The figure shows three views and two pictorial views of one solid part (mm, origin at its lowest corner). Answer the questions. Round coordinates to 2 decimals unless told otherwise and drop trailing zeros. Order: outer loops, then holes, each group sorted by start corner. A loop starts at its lowest first (then second) coordinate and runs counter-clockwise, first axis right, second up. Notation, with made-up numbers: M 48.5,-1.75 L 54.5,-1.75 A26 cw 54.5,30.25 Z; hole C -24.5,52 d3. An arc over 180 degrees is marked long. Return JSON: item names as keys, results as strings.
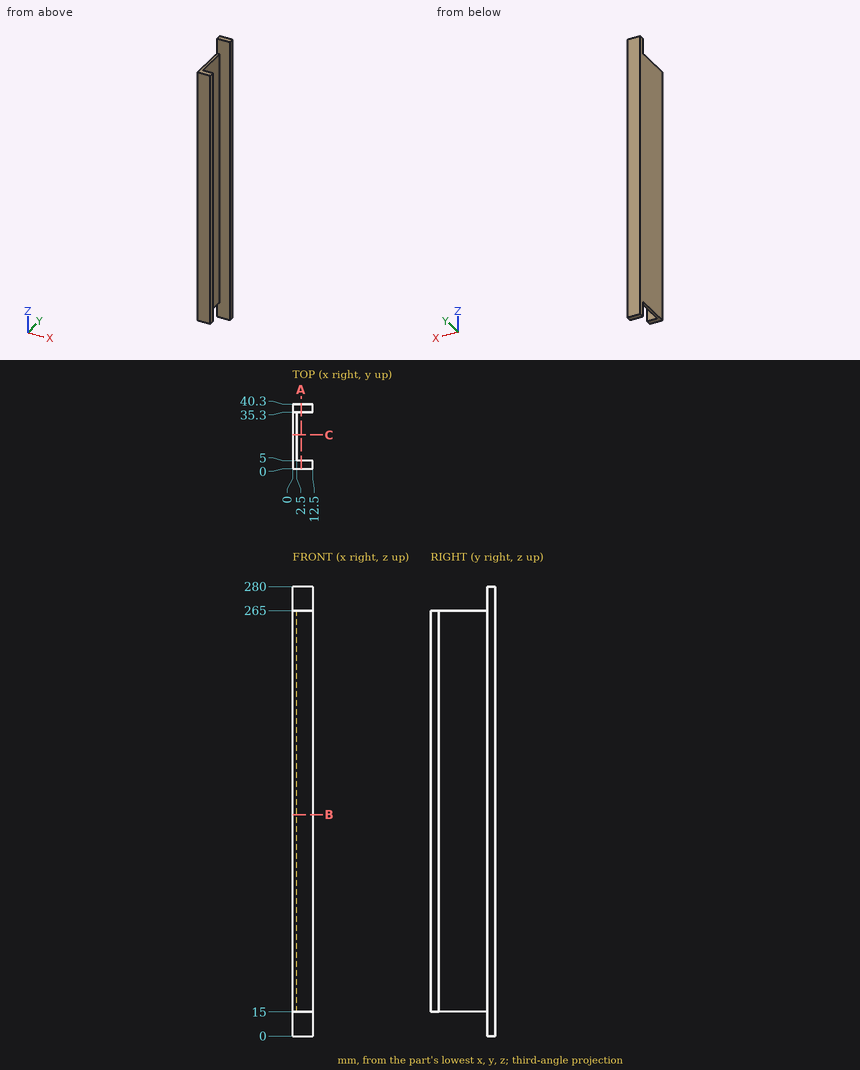
Item 1: Each of these flat-tipped pins is pushed along its axis until it touches: pin 1 (6 mm diameter, centred on y = 27.5, z = 212, fed in from -X); pin 2 (1.5 mm diameter, centred on x = 3.5, y = 28.5, fed in from +Z); pin 3 (10 mm diameter, centred on y = 29.5, z = 150.5, fed in from +X). Where does it stop, or does it pass through?
Output:
{"pin 1": "stops at x = 0", "pin 2": "passes through", "pin 3": "stops at x = 2.5"}
Item 2: Find section B-B (z = 138). Determine the outline of the cut face in (x, y), plus the area to 3 significant figures.
Output:
{"outline": "M 0,0 L 12.5,0 L 12.5,5 L 2.5,5 L 2.5,35.3 L 12.5,35.3 L 12.5,40.3 L 0,40.3 Z", "area": "201 mm^2"}
Item 3: Find section C-C (y = 21). Determine the outline of the cut face in (x, z), plus the area to 3 significant figures.
Output:
{"outline": "M 0,15 L 2.5,15 L 2.5,265 L 0,265 Z", "area": "625 mm^2"}
Item 4: Consider line 1 along Y through (x, z) = (10.5, 174.5); line 2 along X through (y, z) = (23, 247.5); line 3 along Z through (x, y) = (9.5, 3.5). Determine where each line is inside the solid, lowest interval first. Write a range as [from, to].
Output:
{"line 1": "y = [0, 5], [35.3, 40.3]", "line 2": "x = [0, 2.5]", "line 3": "z = [15, 265]"}
Item 5: Find section A-A (x = 5.25). Determine the outline of the cut face in (y, z), plus the area to 3 significant figures.
Output:
{"outline": "M 0,15 L 5,15 L 5,265 L 0,265 Z; M 35.3,0 L 40.3,0 L 40.3,280 L 35.3,280 Z", "area": "2,650 mm^2"}
